Autodesk Inventor part; units mm, degrees
ref_plane "Work Plane1" through (0, 0, -43.05) normal (0, 0, -1) x (0, 1, 0)
ref_plane "YZ Plane" through (0, 0, 0) normal (1, 0, 0) x (0, 1, 0)
ref_plane "XZ Plane" through (0, 0, 0) normal (0, 1, 0) x (-1, 0, 0)
sketch "Sketch1" plane through (0, 0, 0) normal (0, 0, 1) x (1, 0, 0)
  line L0 (0, 0) -> (0, 1.3)
  line L1 (0, 0) -> (17.2, 0)
  line L2 (17.2, 0) -> (17.2, 1.3)
  line L3 (0, 1.3) -> (17.2, 1.3)
  line L4 (-0.2, -0.2) -> (-0.2, 1.5)
  line L5 (17.4, 1.5) -> (17.4, -0.2)
  line L6 (-2.2, 3.5) -> (-2.2, -2.2)
  line L7 (19.4, -2.2) -> (19.4, 3.5)
  line L8 (0.49, 2.4) -> (0.49, 1.65)
  line L9 (0.29, 2.4) -> (0.29, 1.65)
  line L10 (16.69, 2.4) -> (16.69, 1.65)
  line L11 (16.89, 2.4) -> (16.89, 1.65)
  line L12 (16.89, 1.5) -> (16.89, 3.5)
  line L13 (0.29, 1.5) -> (0.29, 3.5)
  line L14 (19.4, 3.5) -> (16.89, 3.5)
  line L15 (0.29, 3.5) -> (-2.2, 3.5)
  line L16 (-0.2, 1.5) -> (0.29, 1.5)
  line L17 (16.89, 1.5) -> (17.4, 1.5)
  line L18 (15.45, -2) -> (0.93, -2)
  line L19 (-2, -2) -> (-2, 3.3)
  line L20 (19.2, 3.3) -> (19.2, -2)
  line L21 (1.13, -0.1) -> (1.13, 0)
  line L22 (0.93, -0.1) -> (0.93, 0)
  line L23 (0.93, 0) -> (0.93, -2)
  line L24 (15.25, -0.1) -> (15.25, 1.4)
  line L25 (15.45, -0.1) -> (15.45, 1.4)
  line L26 (15.45, 1.3) -> (15.45, -2)
  line L27 (-2.2, -2.2) -> (-2.2, -4.2)
  line L28 (-2.2, -4.2) -> (19.4, -4.2)
  line L29 (19.4, -4.2) -> (19.4, -2.2)
  line L30 (17.4, -0.2) -> (15.45, -0.2)
  line L31 (0.93, -0.2) -> (-0.2, -0.2)
  line L32 (0.49, -2.2) -> (1.13, -2.2)
  line L33 (15.25, -2.2) -> (16.89, -2.2)
  line L34 (-2.2, -2.2) -> (-2, -2.2)
  line L35 (-0.2, -2.2) -> (0.29, -2.2)
  line L36 (17.2, -2.2) -> (17.4, -2.2)
  line L37 (19.2, -2.2) -> (19.4, -2.2)
  line L38 (0.29, 3.3) -> (1.13, 3.3)
  line L39 (15.25, 3.3) -> (16.89, 3.3)
  dimension "d2" = 0.2
  dimension "d3" = 0.2
  dimension "d4" = 2
  dimension "d5" = 0.2
  dimension "d6" = 0.2
  dimension "d7" = 2
ref_plane "Work Plane1" through (0, 0, -43.05) normal (0, 0, -1) x (0, 1, 0)
extrude "Extrusion1" add sketch "Sketch1" against normal up to surface (43.05 mm away) contours L23 L18 L26 L30 L5 L17 L12 L11 L14 L7 L29 L28 L27 L6 L15 L13 L9 L16 L4 L31
chamfer "Chamfer1" distance 0.5 angle 45 2 edges at (15.45, -0.2, -21.525) (0.93, -0.2, -21.525)
chamfer "Chamfer2" distance 0.2 angle 45 2 edges at (0.29, 1.5, -21.525) (16.89, 1.5, -21.525)
sketch "Sketch2" plane through (19.4, -4.2, -43.05) normal (0, 0, -1) x (-1, 0, 0)
  line L0 (2.51, 5.9) -> (2.31, 5.7)
  line L1 (2.51, 7.7) -> (2.51, 5.9)
  line L2 (0, 7.7) -> (2.51, 7.7)
  line L3 (0, 0) -> (0, 7.7)
  line L4 (21.6, 0) -> (0, 0)
  line L5 (21.6, 7.7) -> (21.6, 0)
  line L6 (19.11, 7.7) -> (21.6, 7.7)
  line L7 (19.11, 5.9) -> (19.11, 7.7)
  line L8 (19.31, 5.7) -> (19.11, 5.9)
  line L9 (19.6, 5.7) -> (19.31, 5.7)
  line L10 (19.6, 4) -> (19.6, 5.7)
  line L11 (18.97, 4) -> (19.6, 4)
  line L12 (18.47, 3.5) -> (18.97, 4)
  line L13 (18.47, 2.2) -> (18.47, 3.5)
  line L14 (3.95, 2.2) -> (18.47, 2.2)
  line L15 (3.95, 3.5) -> (3.95, 2.2)
  line L16 (3.45, 4) -> (3.95, 3.5)
  line L17 (2, 4) -> (3.45, 4)
  line L18 (2, 5.7) -> (2, 4)
  line L19 (2.31, 5.7) -> (2, 5.7)
  line L20 (0, 5.7) -> (21.6, 5.7)
  point P0 (19.4, 4.2)
extrude "Extrusion2" add sketch "Sketch2" along normal blind 2
sketch "Sketch3" plane through (-2.2, -4.2, 0) normal (0, -1, 0) x (1, 0, 0)
  line L0 (21.6, 0) -> (21.6, -45.05)
  line L1 (21.6, 0) -> (26.6, 0)
  line L2 (28.6, -2) -> (28.6, -43.05)
  line L3 (26.6, -45.05) -> (21.6, -45.05)
  line L4 (28.6, 0) -> (25.6, 0)
  line L5 (25.6, 0) -> (25.6, -45.05)
  line L6 (25.6, 0) -> (25.6, -6)
  line L7 (25.6, -45.05) -> (25.6, -39.05)
  circle A0 centre (25.6, -6) radius 1.5
  circle A1 centre (25.6, -39.05) radius 1.5
  arc A2 (28.6, -2) -> (26.6, 0) centre (26.6, -2) ccw
  arc A3 (26.6, -45.05) -> (28.6, -43.05) centre (26.6, -43.05) ccw
  point P0 (2.2, 0)
  dimension "d18" = 7
  dimension "d19" = 3
  dimension "d20" = 6
  dimension "d21" = 6
  dimension "d22" = 3
  dimension "d23" = 3
  dimension "d24" = 2
extrude "Extrusion3" add sketch "Sketch3" against normal blind 2 contours L1 L5 A0 A1 L3 L0 | L1 A2 L2 A3 L3 L5 A1 A0
chamfer "Chamfer3" distance 1 angle 45 1 edges at (19.4, -2.2, -22.525)
sketch "Sketch4" plane through (26.4, -4.2, -2) normal (1, 0, 0) x (0, 0, -1)
  line L0 (0, 2) -> (41.05, 2)
  line L1 (20.525, 2) -> (20.525, 7.7)
  line L2 (-2, 7.7) -> (43.05, 7.7)
  line L3 (22.025, 7.7) -> (19.025, 7.7)
  line L4 (19.025, 7.7) -> (19.025, 2)
  line L5 (19.025, 2) -> (22.025, 2)
  line L6 (22.025, 2) -> (22.025, 7.7)
  line L7 (22.025, 7.7) -> (19.025, 2) construction
  line L8 (19.025, 7.7) -> (22.025, 2) construction
  point P0 (-2, 4.2)
  point P1 (20.525, 4.85)
  point P2 (19.025, 7.7)
  point P3 (22.025, 2)
  point P4 (22.025, 7.7)
  dimension "d30" = 3
extrude "Extrusion4" add sketch "Sketch4" against normal up to surface (7 mm away)
fillet "Fillet1" radius 4 1 edges at (26.4, 3.5, -22.525)
chamfer "Chamfer4" distance 1 angle 45 2 edges at (23.4, -2.2, -21.025) (23.4, -2.2, -24.025)
properties part number "relay_case_3DPrint"
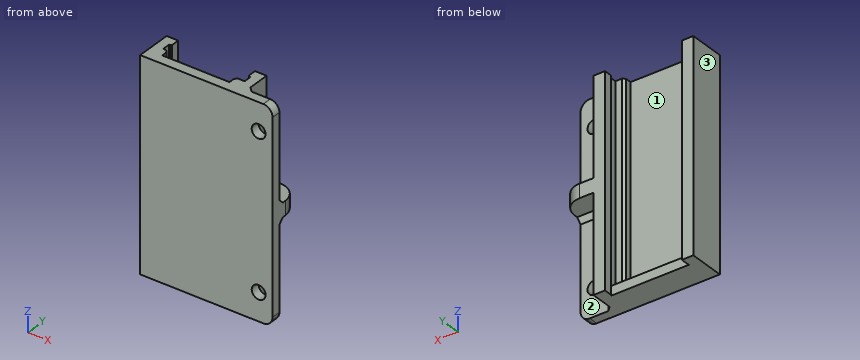
Here's how the part is built. I have some questions about the finished solid (model axes, mm). Face numbers are marked on the shaded views. A direction names the side the tool comes from. Coordinates: 2 decimals unless noted, no trailing zeros. Write each loop counter-clockwise with the first axis right and the second up, starting at its lowest first coordinate (ties: lowest second). Pieces come first, ordered by that corner, then holes. Notation, with made-up numbers: (57, -12) -> (65, -12) arc R22 ccw to (65, 7) -> close; hole circle Ø9 at (2, 51). An arc over 180 degrees is marked (long way). Use a Markdown table: item, result. Add a question column.
(1) Please list where these lines run through material, in increasing order: line 1 (Z direction, x = 23.4, y = -2.55); line 2 (X direction, y = 2, z = -31); line 3 (X direction, y = 0, z = -20).
(2) For the marked faces 1, 2 and 3, which set-ups out of +Z, -Z, +X, -X, +Y, -Y let a thin tool reach every point of the face, with its end or its side?
(3) If we section it at A-A, the plane z = -39.05: Write out the boundary of the cut face in (x, y).
(4) If we section it at B-B, the plane x = 23.4: Write out the boundary of the cut face in (y, z) (3 decimals), and give its area (3 significant figures).
(5) If we section it at D-D, the plane z = -12.5: Write out the boundary of the cut face in (x, y), and give its area (3 significant figures).
(6) If we section it at C-C, the plane y = 2.5: Write out the boundary of the cut face in (x, z) (3 decimals), and give its area (3 significant figures).
(7) I'm going to push flat-ended pins straight in: P1, Ø4.5, axis at x = 6, z = -26, coming from the +Y side; P2, Ø3.5, axis at x = 23.4, z = -39.05, coming from the +Y side; P3, Ø1.4, axis at y = 2, z = -22.5, coming from the +X side. Where does each tip first touch, or does it pass through?
Outcome:
| question | item | result |
|---|---|---|
| 1 | line 1 | z = -45.05 to -40.55, -37.55 to -7.5, -4.5 to 0 |
| 1 | line 2 | x = -2.2 to 0.29, 16.89 to 19.4 |
| 1 | line 3 | x = -2.2 to -0.2, 17.4 to 19.4 |
| 2 | face 1 | +Z, +Y |
| 2 | face 2 | -Z, +X, +Y |
| 2 | face 3 | +Z, -Z, -X, +Y, -Y |
| 3 | outline | (-2.2, -4.2) -> (21.9, -4.2) -> (21.9, -2.2) -> (20.4, -2.2) -> (19.4, -1.2) -> (19.4, 3.5) -> (16.89, 3.5) -> (16.89, 1.7) -> (17.09, 1.5) -> (17.4, 1.5) -> (17.4, -0.2) -> (15.95, -0.2) -> (15.45, -0.7) -> (15.45, -2) -> (0.93, -2) -> (0.93, -0.7) -> (0.43, -0.2) -> (-0.2, -0.2) -> (-0.2, 1.5) -> (0.09, 1.5) -> (0.29, 1.7) -> (0.29, 3.5) -> (-2.2, 3.5) -> close; (24.9, -4.2) -> (26.4, -4.2) -> (26.4, -2.2) -> (24.9, -2.2) -> close |
| 4 | outline | (-4.2, -45.05) -> (-2.2, -45.05) -> (-2.2, -40.55) -> (-4.2, -40.55) -> close; (-4.2, -37.55) -> (-2.2, -37.55) -> (-2.2, -25.025) -> (-1.2, -24.025) -> (3.373, -24.025) -> (3.373, -21.025) -> (-1.2, -21.025) -> (-2.2, -20.025) -> (-2.2, -7.5) -> (-4.2, -7.5) -> close; (-4.2, -4.5) -> (-2.2, -4.5) -> (-2.2, 0) -> (-4.2, 0) -> close |
| 4 | area | 95.8 mm^2 |
| 5 | outline | (-2.2, -4.2) -> (26.4, -4.2) -> (26.4, -2.2) -> (20.4, -2.2) -> (19.4, -1.2) -> (19.4, 3.5) -> (16.89, 3.5) -> (16.89, 1.7) -> (17.09, 1.5) -> (17.4, 1.5) -> (17.4, -0.2) -> (15.95, -0.2) -> (15.45, -0.7) -> (15.45, -2) -> (0.93, -2) -> (0.93, -0.7) -> (0.43, -0.2) -> (-0.2, -0.2) -> (-0.2, 1.5) -> (0.09, 1.5) -> (0.29, 1.7) -> (0.29, 3.5) -> (-2.2, 3.5) -> close |
| 5 | area | 91.3 mm^2 |
| 6 | outline | (-2.2, -45.05) -> (0.29, -45.05) -> (0.29, 0) -> (-2.2, 0) -> close; (16.89, -45.05) -> (19.4, -45.05) -> (19.4, -24.025) -> (25.046, -24.025) -> (25.046, -21.025) -> (19.4, -21.025) -> (19.4, 0) -> (16.89, 0) -> close |
| 6 | area | 242 mm^2 |
| 7 | P1 | stops at y = -2 |
| 7 | P2 | stops at y = -2.2 |
| 7 | P3 | stops at x = 25.97 |
